The listing builds one solid part. Answer for the finished solid, in the listing's coordinates (mm). Face numbers are marked on the shaded views. A direction names the side the tool comes from. Coordinates: 2 decimals unless noted, no trailing zeros. Loops run counter-clockwise (first coordinate to the right, second up) from the corner with the lowest first, then second, coordinate; pieces in that order, holes last. Notation, with made-up numbers: M 17,80.25 L 45,80.25 A9 cw 45,97.25 Z; hole C 56.25,16.5 d10. An arc over 180 degrees is marked long. Return JSON: item names as keys, results as strings. Group by question number.
1. Section B-B (x = 20.32) is taken. Write down the section's boundary in (y, z) (3 decimals).
2. Given P1, Ø6, axis at y = 68, z = 12, coming from the +X side (3 decimals); P2, Ø1.5, axis at x = 3.5, y = 66, coming from the -Z side; P3, Ø7.5, axis at x = 12.065, y = 34.925, coming from the +Z side (3 decimals), each flat-ended and moving along its own axis, determine where each tip first touches the part or whether it passes through.
3. Section D-D (z = 13.5) is taken. Write down the section's boundary in (x, y) (3 decimals), then the cut area to 3 significant figures.
4. Section A-A (y = 12.7) is taken. Write down the section's boundary in (x, z) (3 decimals).
5. Section C-C (z = 25.5) is taken. Write down the section's boundary in (x, y) (3 decimals).
6. Which of the six approach directions +Z, -Z, +X, -X, +Y, -Y give full straight-line access (tool end or side, diameter ignored) to the marked faces 1 and 2?
7. Straight lines are drawn through the part: L1, parallel to Y at x = 20.32, z = 2.5; L2, parallel to X at y = 44, z = 34 (3 decimals). For each, find the intervals that lie inside material, in ascending order. Write a range as from..to.
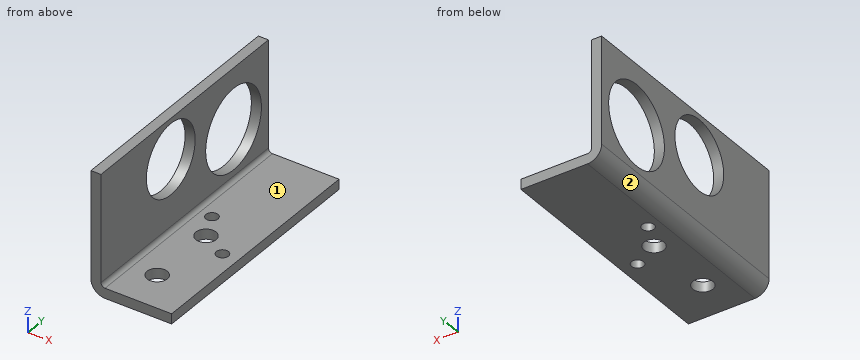
Autodesk Inventor part; units mm, degrees
ref_plane "YZ Plane" through (0, 0, 0) normal (1, 0, 0) x (0, 1, 0)
ref_plane "XZ Plane" through (0, 0, 0) normal (0, 1, 0) x (-1, 0, 0)
ref_plane "XY Plane" through (0, 0, 0) normal (0, 0, 1) x (1, 0, 0)
sketch "Sketch1" plane through (0, 0, 0) normal (0, 0, 1) x (1, 0, 0)
  line L0 (0, 0) -> (25.4, 0)
  line L1 (25.4, 0) -> (25.4, 76.2)
  line L2 (25.4, 76.2) -> (0, 76.2)
  line L3 (0, 76.2) -> (0, 0)
  dimension "d0" = 25.4
  dimension "d1" = 76.2
extrude "Plate1" add sketch "Sketch1" along normal blind 3.175
sketch "Sketch2" plane through (3.175, 0, 0) normal (-1, 0, 0) x (0, -1, 0)
  line L0 (-76.2, 0) -> (0, 0)
  line L1 (0, 0) -> (0, 38.1)
  line L2 (0, 38.1) -> (-76.2, 38.1)
  line L3 (-76.2, 38.1) -> (-76.2, 0)
edge flange "Flange1" height 38.1 angle 90 thickness 3.175 bend radius 1.27 thickness toward (-1, 0, 0) relief tear relief width 3.175 relief depth 1.5875 edges at (0, 38.1, 3.175) wall of the first edge with corners at (3.175, 76.2, 0) (3.175, 0, 0) (3.175, 0, 38.1) (3.175, 76.2, 38.1)
bend "Bend1"
corner "Corner1"
sketch "Sketch3" plane through (0, 0, 38.1) normal (-1, 0, 0) x (0, 0, 1)
  line L0 (0, 0) -> (-33.655, 0)
  line L1 (0, 76.2) -> (0, 0)
  line L2 (-33.655, 76.2) -> (0, 76.2)
  circle A0 centre (-19.05, 60.325) radius 12.7
  circle A1 centre (-12.7, 31.75) radius 11.1125
  point P0 (-38.1, 0)
  dimension "d13" = 25.4
  dimension "d14" = 22.225
  dimension "d15" = 15.875
  dimension "d16" = 19.05
  dimension "d17" = 12.7
  dimension "d18" = 31.75
extrude "Cut1" cut sketch "Sketch3" against normal blind 3.175
sketch "Sketch4" plane through (0, 0, 3.175) normal (0, 0, 1) x (1, 0, 0)
  line L0 (4.445, 76.2) -> (4.445, 0)
  line L1 (25.4, 76.2) -> (25.4, 0)
  circle A0 centre (-69.6884, -88.0779) radius 3.3782 construction
  circle A1 centre (-79.6289, 46.8501) radius 3.3782 construction
  circle A2 centre (-113.1559, 49.7834) radius 3.3782 construction
  circle A3 centre (-43.9071, -66.4449) radius 3.3782 construction
  line L2 (-118.5182, 63.001) -> (-315.8997, 80.2697) construction
  arc A4 (-315.8997, 80.2697) -> (-318.1134, 54.9663) centre (74.9912, 33.3226) ccw construction
  line L3 (-318.1134, 54.9663) -> (38.1, 23.8017) construction
  arc A5 (38.1, 23.8017) -> (42.1314, 14.0393) centre (74.9912, 33.3226) ccw construction
  line L4 (42.1314, 14.0393) -> (-230.643, -214.8455) construction
  arc A6 (-230.643, -214.8455) -> (-226.6005, -219.7429) centre (74.9912, 33.3226) ccw construction
  line L5 (-226.6005, -219.7429) -> (-222.5188, -224.6072) construction
  line L6 (-222.5188, -224.6072) -> (50.2948, 4.3106) construction
  arc A7 (50.2948, 4.3106) -> (55.7079, 66.1824) centre (74.9912, 33.3226) ccw construction
  line L7 (55.7079, 66.1824) -> (15.7878, 113.7573) construction
  arc A8 (-3.434, 116.9073) -> (15.7878, 113.7573) centre (29.7432, 259.139) ccw construction
  line L8 (-3.434, 116.9073) -> (-110.1078, 141.7901) construction
  line L9 (-110.1078, 141.7901) -> (-116.0889, 251.1642) construction
  arc A9 (-115.8532, 270.641) -> (-116.0889, 251.1642) centre (29.7432, 259.139) ccw construction
  line L10 (-115.8532, 270.641) -> (-173.2099, 338.996) construction
  line L11 (-173.2099, 338.996) -> (-178.0743, 334.9143) construction
  arc A10 (-178.0743, 334.9143) -> (-182.9057, 330.7934) centre (74.9912, 33.3226) ccw construction
  line L12 (-182.9057, 330.7934) -> (-129.6946, 267.3788) construction
  line L13 (-129.6946, 267.3788) -> (-118.5182, 63.001) construction
  circle A11 centre (-173.9926, 330.0499) radius 3.3782 construction
  circle A12 centre (-141.339, 291.1349) radius 3.3782 construction
  line L14 (-105.7381, 61.8829) -> (-109.3854, 128.5807) construction
  line L15 (-109.3854, 128.5807) -> (10.1717, 100.6927) construction
  line L16 (10.1717, 100.6927) -> (45.9792, 58.019) construction
  arc A13 (45.9792, 58.019) -> (40.3138, 49.105) centre (74.9912, 33.3226) ccw construction
  line L17 (40.3138, 49.105) -> (-105.7381, 61.8829) construction
  circle A14 centre (74.9912, 33.3226) radius 9.5 construction
  circle A15 centre (-310.4012, 72.216) radius 3.3782 construction
  circle A16 centre (-311.3, 61.9429) radius 3.3782 construction
  circle A17 centre (-259.7945, 67.7885) radius 3.3782 construction
  circle A18 centre (-260.6933, 57.5153) radius 3.3782 construction
  circle A19 centre (-221.7361, -215.6611) radius 3.3782 construction
  circle A20 centre (-182.821, -183.0075) radius 3.3782 construction
  circle A21 centre (-32.0252, -56.4748) radius 3.3782 construction
  circle A22 centre (-139.0416, -146.2722) radius 3.3782 construction
  circle A23 centre (-63.4799, 51.8115) radius 3.3782 construction
  circle A24 centre (-64.5868, 39.1599) radius 3.3782 construction
  circle A25 centre (-202.7203, 63.9935) radius 3.3782 construction
  circle A26 centre (-203.8271, 51.3418) radius 3.3782 construction
  circle A27 centre (20.32, 30.4566) radius 1.905
  circle A28 centre (8.255, 43.1566) radius 1.905
  line L18 (25.4, 0) -> (4.445, 0)
  line L19 (4.445, 76.2) -> (25.4, 76.2)
  line L20 (12.065, 76.2) -> (12.065, 0) construction
  circle A29 centre (12.065, 12.7) radius 3.175
  circle A30 centre (12.065, 34.925) radius 3.175
  point P0 (0, 0)
  dimension "d21" = 3.81
  dimension "d22" = 5.08
  dimension "d23" = 5.08
  dimension "d24" = 12.7
  dimension "d25" = 3.81
  dimension "d28" = 7.62
  dimension "d29" = 6.35
  dimension "d30" = 12.7
  dimension "d31" = 22.225
extrude "Cut2" cut sketch "Sketch4" against normal blind 3.175 contours A27 | A28 | A29 | A30
equation "\"d19\" = Thickness"
equation "\"d26\" = Thickness"
equation "\"d3\" = BendReliefWidth"
equation "\"d4\" = BendReliefDepth"
equation "\"d5\" = MinimumRemnant"
equation "\"d6\" = BendRadius"
equation "\"d10\" = CornerReliefSize"
equation "\"d11\" = GapSize"
equation "\"d12\" = JacobiRadiusSize"
equation "\"BendRadius\" = Thickness"
equation "\"BendReliefWidth\" = Thickness"
equation "\"BendReliefDepth\" = 0.5 * Thickness"
equation "\"CornerReliefSize\" = 4 * Thickness"
equation "\"MinimumRemnant\" = 2 * Thickness"
equation "\"TransitionRadius\" = BendRadius"
equation "\"JacobiRadiusSize\" = BendRadius"
equation "\"GapSize\" = Thickness"
equation "\"d2\" = BendRadius"
properties part number "Shooter Magnetic Sensor Mount Bracket" material "Aluminum 6061"
Worked out:
{
 "1": {"outline": "M 0,0 L 28.552,0 L 28.552,3.175 L 0,3.175 Z; M 32.362,0 L 76.2,0 L 76.2,3.175 L 32.362,3.175 Z"},
 "2": {"P1": "x = 3.175", "P2": "z = 0", "P3": "z = 3.175"},
 "3": {"outline": "M 0,0 L 3.175,0 L 3.175,48.902 L 0,48.902 Z; M 0,71.748 L 3.175,71.748 L 3.175,76.2 L 0,76.2 Z", "area": "169 mm^2"},
 "4": {"outline": "M 0,4.445 A4.445 ccw 4.445,0 L 8.89,0 L 8.89,3.175 L 4.445,3.175 A1.27 cw 3.175,4.445 L 3.175,38.1 L 0,38.1 Z; M 15.24,0 L 25.4,0 L 25.4,3.175 L 15.24,3.175 Z"},
 "5": {"outline": "M 0,0 L 3.175,0 L 3.175,20.638 L 0,20.638 Z; M 0,42.862 L 3.175,42.862 L 3.175,49.385 L 0,49.385 Z; M 0,71.265 L 3.175,71.265 L 3.175,76.2 L 0,76.2 Z"},
 "6": {"face 1": "+Z, +X, +Y, -Y", "face 2": "-Z, -X, +Y, -Y"},
 "7": {"L1": "0..28.55, 32.36..76.2", "L2": "0..3.175"}
}
